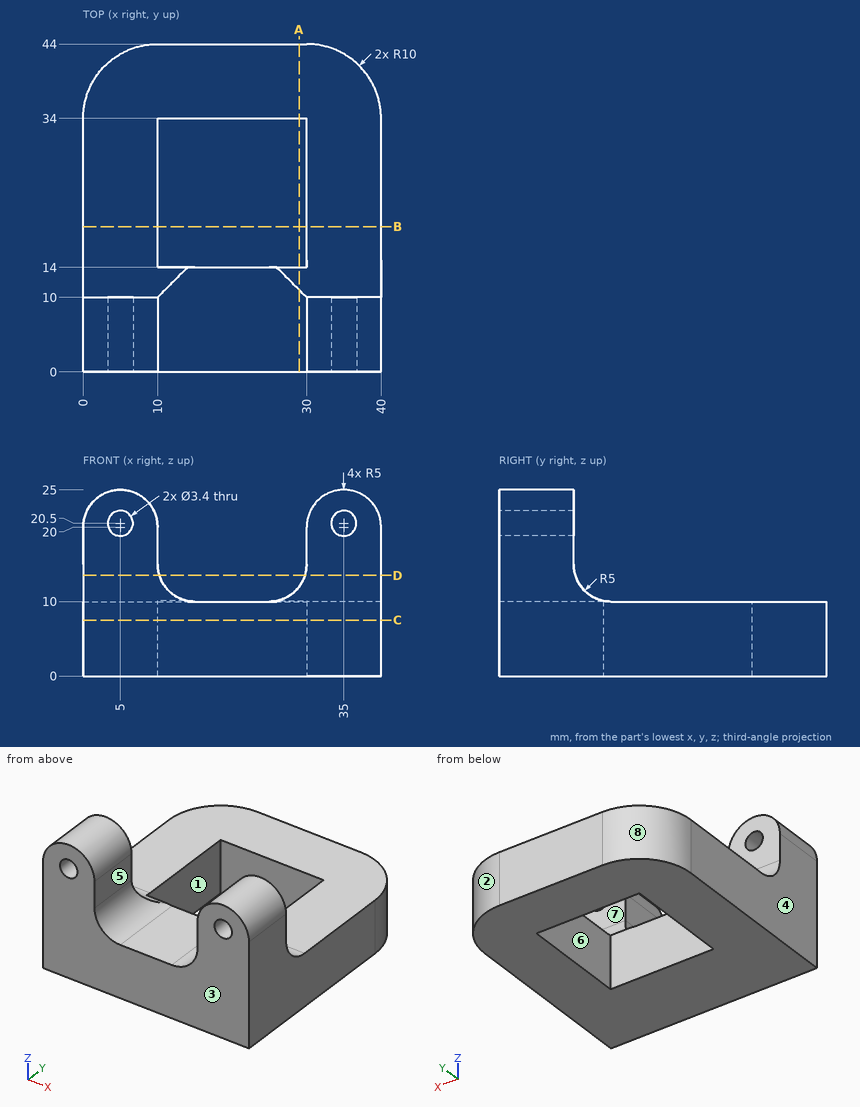
Design review of the part shown in the three views and the two pictorial views. Dimensions are in mm from the part's minimum x, y and z. A direction names the side the tool comes from. Round coordinates to 2 decimals unless told otherwise and drop trailing zeros. Loops run counter-clockwise (first coordinate to the right, second up) from the corner with the lowest first, then second, coordinate; pieces in that order, holes last.
Q1. Add section A-A on x = 29. Write out the cut boundary in (y, z), plus the area to 3 significant figures.
Result sheet:
outline: (0, 0) - (14, 0) - (14, 10.1) arc R5 cw to (11, 12) - (0, 12) - close; (34, 0) - (44, 0) - (44, 10) - (34, 10) - close
area: 264 mm2
Q2. Add section C-C on z = 7.5. Write out the cut boundary in (x, y), plus the area to 3 significant figures.
Result sheet:
outline: (0, 0) - (40, 0) - (40, 34) arc R10 ccw to (30, 44) - (10, 44) arc R10 ccw to (0, 34) - close; hole (10, 14) - (30, 14) - (30, 34) - (10, 34) - close
area: 1,320 mm2
Q3. Add section B-B on y = 19.5. Write out the cut boundary in (x, z), plus the area to 3 significant figures.
Result sheet:
outline: (0, 0) - (10, 0) - (10, 10) - (0, 10) - close; (30, 0) - (40, 0) - (40, 10) - (30, 10) - close
area: 200 mm2
Q4. Insertion check: pin 1 Ø3 at (x, z) = (36, 21.5) entering from +Y; pin 2 Ø12 at (x, y) = (34, 33) entering from +Z. Each pin has a flat end and moves straight along its axis. Give the tip position at first contact, or say it passes through.
Result sheet:
pin 1: stops at y = 10
pin 2: stops at z = 10
Q5. Machinability: for the marked faces 5, 6, 7 and 8, which of the approach directions +Z, -Z, +X, -X, +Y, -Y give a long, thin tool a straight path to every point of the face, cutting with its end or side? Answer none if there is none.
Result sheet:
face 5: +Z, +Y, -Y
face 6: +Z, -Z
face 7: +Z, +X, -X, +Y
face 8: +Z, -Z, -X, +Y
Q6. To check wall thickness, follow line 1 along Z through (x, y) = (5, 6); line 2 along X through (y, z) = (20, 9); line 3 along X through (y, z) = (6, 20.5). State the ranges of each line that lie inside material, in increasing order.
Result sheet:
line 1: z = 0 to 18.8, 22.2 to 25
line 2: x = 0 to 10, 30 to 40
line 3: x = 0.03 to 3.3, 6.7 to 9.97, 30.03 to 33.3, 36.7 to 39.97
Q7. Add section D-D on z = 13.5. Write out the cut boundary in (x, y).
Result sheet:
outline: (0, 0) - (10.23, 0) - (10.23, 10.23) - (0, 10.23) - close; (29.77, 0) - (40, 0) - (40, 10.23) - (29.77, 10.23) - close
Q8. Mouldability with a two-part tool opening along Y and no side actions: class the marked faces 1, 2, 3 and 4 as +Y half, -Y half, draft (parallel to the pull), parting line (faces both ways), or undercut.
Result sheet:
face 1: undercut
face 2: +Y half
face 3: -Y half
face 4: draft
